Could you check a few things on this model? Use its own coordinates, in mm. A direction names the side the tool comes from. Coordinates: 2 decimals unless noted, no trailing zeros. Loops run counter-clockwise (first coordinate to the right, second up) from the corner with the lowest first, then second, coordinate; pieces in that order, holes last.
1) Imagine slicing it at A-A on y = 77. Please give me the cut outline in (x, z), plus the area to 3 significant figures.
2) For faces 1 (the face through (-6, 80, 17.5)), 2 (the face through (-10.25, 75, 6)), 3 (the face through (-1, 70, 12.5)), which set-ups out of +Z, -Z, +X, -X, +Y, -Y let a thin tool reach every point of the face, with its end or its side?
3) Will these pins go through, and if not, where does the flat tip stop? P1, Ø2.5, axis at x = -5, y = 97.5, coming from the +Z side; P2, Ø0.6, axis at x = -1, y = 77.5, coming from the -Z side; P3, Ø2, axis at y = 22, z = 19.5, coming from the +X side.
4) If I drill on line 1 along X through (y, z) = (13.5, 1.1) (3 decimals); line 2 along Y through (x, z) = (-7.25, 5.25); line 3 along X through (y, z) = (13.5, 2.1) (3 decimals), over which ranges is the centre line in solid material (lowest first)?
```python
from build123d import *

# Parameters (mm, degrees)
SKETCH1_W           = 100
SKETCH1_H           = 11.75
BOSS_EXTRUDE1_DEPTH = 17.5
SKETCH5_R           = 2.65
CUT_EXTRUDE2_DEPTH  = 103.197419243
SKETCH4_W           = 50
SKETCH4_H           = 12.5
SKETCH4_R           = 2.65
CUT_EXTRUDE3_DEPTH  = 1.5
BOSS_EXTRUDE3_DEPTH = 0.5
BOSS_EXTRUDE2_DEPTH = 12.75
CUT_EXTRUDE4_DEPTH  = 105.302744451
FILLET4_R           = 1
FILLET3_R           = 1
CUT_EXTRUDE5_REACH  = 100.641
CUT_EXTRUDE7_REACH  = 106.363
SKETCH13_W          = 5
SKETCH13_H          = 5
FILLET5_R           = 0.5
CUT_EXTRUDE6_DEPTH  = 5
CHAMFER1_SIZE       = 3
CHAMFER1_SIZE2      = 0.262465991
FILLET6_R           = 1


with BuildPart() as part:
    # Sketch1 → Boss-Extrude1 (new body)
    with BuildSketch(Plane(origin=(0, 0, 0), x_dir=(0, 1, 0), z_dir=(0, 0, 1))):
        with Locations((50, 5.875)):
            Rectangle(SKETCH1_W, SKETCH1_H)
    extrude(amount=BOSS_EXTRUDE1_DEPTH)

    # Sketch5 → Cut-Extrude2 (cut, through all)
    with BuildSketch(Plane.YZ):
        with Locations(Location((70, 5, 0), (0, 0, 270))):
            Circle(SKETCH5_R)
    extrude(amount=-CUT_EXTRUDE2_DEPTH, mode=Mode.SUBTRACT)

    # Sketch4 → Cut-Extrude3 (cut)
    with BuildSketch(Plane.YZ):
        with Locations((75, 6.25)):
            Rectangle(SKETCH4_W, SKETCH4_H)
        with Locations(Location((70, 5, 0), (0, 0, 270))):
            Circle(SKETCH4_R, mode=Mode.SUBTRACT)
    cut_extrude3 = extrude(amount=-CUT_EXTRUDE3_DEPTH, mode=Mode.SUBTRACT)

    # Mirror1: Cut-Extrude3 across plane
    add(cut_extrude3.mirror(Plane(origin=(-5.875, 0, 0), x_dir=(0, 0, 1), z_dir=(1, 0, 0))), mode=Mode.SUBTRACT)

    # Sketch9 → Boss-Extrude3 (add)
    with BuildSketch(Plane.YZ):
        Polygon((0, 17.5), (50, 17.5), (100, 17.5), (100, 12.5), (50, 12.5), (50, 0), (0, 0), align=None)
    boss_extrude3 = extrude(amount=BOSS_EXTRUDE3_DEPTH)

    # Mirror4: Boss-Extrude3 across plane
    add(boss_extrude3.mirror(Plane(origin=(-5.875, 0, 0), x_dir=(0, 0, 1), z_dir=(1, 0, 0))))

    # Sketch6 → Boss-Extrude2 (add)
    with BuildSketch(Plane.YZ.offset(0.5)):
        Polygon((4.75, 27), (0, 17.5), (70, 17.5), (70, 25.469208211), align=None)
    extrude(amount=-BOSS_EXTRUDE2_DEPTH)

    # Sketch7 → Cut-Extrude4 (cut, symmetric)
    with BuildSketch(Plane(origin=(0, 100, 0), x_dir=(-1, 0, 0), z_dir=(0, 1, 0))):
        Polygon((-15.35357036, -50.966517558), (-0.5, 15), (2.202019917, 27), (17.055590277, 92.966517558), (-114.877444838, 122.673658277), (-147.286605475, -21.259376838), align=None)
    cut_extrude4 = extrude(amount=CUT_EXTRUDE4_DEPTH, both=True, mode=Mode.SUBTRACT)

    # Mirror3: Cut-Extrude4 across plane
    add(cut_extrude4.mirror(Plane(origin=(-5.875, 0, 0), x_dir=(0, 0, 1), z_dir=(1, 0, 0))), mode=Mode.SUBTRACT)

    # Fillet4
    fillet4_edges = [part.edges().sort_by_distance(p)[0] for p in [
        (-2.029677005, 37.375, 26.234604106),
        (-1.132470367, 2.375, 22.25),
        (-5.875, 0, 17.5),
        (-9.720322995, 37.375, 26.234604106),
        (-10.617529633, 2.375, 22.25),
    ]]
    fillet(fillet4_edges, radius=FILLET4_R)

    # Fillet3
    # the kernel refuses this fillet: 1 mm, written as the material it takes off along each edge
    with BuildSketch(Plane(origin=(-12.25, 0, -2.5), x_dir=(1, 0, 0), z_dir=(0, 0, 1))) as fillet3_piece_1:
        with BuildLine():
            CenterArc((FILLET3_R, FILLET3_R), FILLET3_R, 180, 90)
            Line((0, FILLET3_R), (0, 0))
            Line((0, 0), (FILLET3_R, 0))
        make_face()
    extrude(amount=20, mode=Mode.SUBTRACT)
    with BuildSketch(Plane(origin=(0.5, 0, -2.5), x_dir=(-1, 0, 0), z_dir=(0, 0, 1))) as fillet3_piece_2:
        with BuildLine():
            CenterArc((FILLET3_R, -FILLET3_R), FILLET3_R, 90, 90)
            Line((0, -FILLET3_R), (0, 0))
            Line((0, 0), (FILLET3_R, 0))
        make_face()
    extrude(amount=20, mode=Mode.SUBTRACT)

    # Sketch11 → Cut-Extrude5 (cut, up to next)
    with BuildSketch(Plane(origin=(0.5, 95.880843205, 19.349640389), x_dir=(0, 0, 1), z_dir=(1, 0, 0)), mode=Mode.PRIVATE) as cut_extrude5_sk1:
        with BuildLine():
            Line((-6.849640389, 0.880843205), (-1.849640389, 0.880843205))
            ThreePointArc((-1.849640389, 0.880843205), (0.650359611, 3.380843205), (-1.849640389, 5.880843205))
            Line((-1.849640389, 5.880843205), (-6.849640389, 5.880843205))
            ThreePointArc((-6.849640389, 5.880843205), (-9.349640389, 3.380843205), (-6.849640389, 0.880843205))
        make_face()
    cut_extrude5_tool1 = extrude(cut_extrude5_sk1.sketch, amount=-CUT_EXTRUDE5_REACH, mode=Mode.PRIVATE) & part.part
    add(cut_extrude5_tool1.solids().sort_by_distance((0.5, 92.5, 15))[0], mode=Mode.SUBTRACT)

    # Sketch13 → Cut-Extrude7 (cut, up to next)
    with BuildSketch(Plane.YZ.offset(0.5), mode=Mode.PRIVATE) as cut_extrude7_sk1:
        with Locations((97.5, 15)):
            Rectangle(SKETCH13_W, SKETCH13_H)
    cut_extrude7_tool1 = extrude(cut_extrude7_sk1.sketch, amount=-CUT_EXTRUDE7_REACH, mode=Mode.PRIVATE) & part.part
    add(cut_extrude7_tool1.solids().sort_by_distance((0.5, 97.5, 15))[0], mode=Mode.SUBTRACT)

    # Fillet5
    fillet5_edges = [part.edges().sort_by_distance(p)[0] for p in [
        (-5.875, 95, 12.5),
        (-5.875, 90, 17.5),
    ]]
    fillet(fillet5_edges, radius=FILLET5_R)

    # Sketch12 → Cut-Extrude6 (cut)
    with BuildSketch(Plane(origin=(0, 0, 0), x_dir=(1, 0, 0), z_dir=(0, 0, -1))):
        with BuildLine():
            ThreePointArc((-2.675, -13.5), (-3.6122583, -11.2372583), (-5.875, -10.3))
            Line((-5.875, -10.3), (-5.875, -10.55))
            ThreePointArc((-5.875, -10.55), (-3.789034995, -11.414034995), (-2.925, -13.5))
            Line((-2.925, -13.5), (-2.675, -13.5))
        make_face()
        with BuildLine():
            Line((-5.875, -10.55), (-5.875, -10.3))
            ThreePointArc((-5.875, -10.3), (-8.1377417, -15.7627417), (-2.675, -13.5))
            Line((-2.675, -13.5), (-2.925, -13.5))
            ThreePointArc((-2.925, -13.5), (-7.960965005, -15.585965005), (-5.875, -10.55))
        make_face()
    extrude(amount=-CUT_EXTRUDE6_DEPTH, mode=Mode.SUBTRACT)

    # Chamfer1
    chamfer1_edges = [part.edges().sort_by_distance(p)[0] for p in [
        (-5.875, 16.45, 0),
    ]]
    chamfer1_side = [part.faces().sort_by_distance(p)[0] for p in [
        (-5.875, 16.45, 2.5),
    ]]
    chamfer(chamfer1_edges, length=CHAMFER1_SIZE, length2=CHAMFER1_SIZE2, reference=chamfer1_side[0])

    # Fillet6
    fillet6_edges = [part.edges().sort_by_distance(p)[0] for p in [
        (-5.875, 16.187534009, 0),
    ]]
    fillet(fillet6_edges, radius=FILLET6_R)


solid = part.part
```
Filled in:
1. outline: (-12.25, 12.5) - (-10.25, 12.5) - (-10.25, 0) - (-1.5, 0) - (-1.5, 12.5) - (0.5, 12.5) - (0.5, 15) - (-0.06, 17.5) - (-11.69, 17.5) - (-12.25, 15) - close
1. area: 172 mm2
2. face 1: +Z, +X, -X, +Y
2. face 2: -Z, -X, +Y
2. face 3: -Z, +X, +Y
3. P1: stops at z = 12.5
3. P2: stops at z = 12.5
3. P3: stops at x = -0.29
4. line 1: x = -12.25 to -9.075, -8.659 to -3.091, -2.675 to 0.5
4. line 2: y = 0 to 67.36, 72.64 to 100
4. line 3: x = -12.25 to -9.075, -8.746 to -3.004, -2.675 to 0.5
